The model under review builds one solid part; all positions refer to its coordinate system, in mm. A direction names the side the tool comes from. Give positions to 0.01 mm unless a question says otherwise; leave off trailing zeros. Write item = value, one per line.
```python
from build123d import *

# Parameters (mm, degrees)
F0_W      = 100
F0_H      = 100
F1_DEPTH  = 50
F2_R      = 42.5
F3_DEPTH  = 15
F4_R      = 42.5
F5_DEPTH  = 15
F6_R      = 42.5
F7_DEPTH  = 15
F8_R      = 42.5
F9_DEPTH  = 15
F10_R     = 30
F11_DEPTH = 10
F12_R     = 30
F13_DEPTH = 10
F14_R     = 30
F15_DEPTH = 10
F16_R     = 30
F17_DEPTH = 10
F18_R     = 20
F19_DEPTH = 10
F20_R     = 20
F21_DEPTH = 10
F22_R     = 20
F23_DEPTH = 10
F24_R     = 20
F25_DEPTH = 10
F26_R     = 12.5
F27_DEPTH = 10
F28_R     = 12.5
F29_DEPTH = 10
F30_R     = 12.5
F31_DEPTH = 65.001
F32_R     = 12.5
F33_DEPTH = 65.001
F34_R     = 42.5
F35_DEPTH = 15
F36_R     = 30
F37_DEPTH = 10
F38_R     = 20
F39_DEPTH = 10
F40_R     = 12.5
F41_DEPTH = 10
F42_R     = 42.5
F43_DEPTH = 15
F44_R     = 30
F45_DEPTH = 10
F46_R     = 20
F47_DEPTH = 10
F48_R     = 12.5
F49_DEPTH = 65.001


with BuildPart() as f1:
    # F0 (on Front) → F1 (new body, symmetric)
    with BuildSketch(Plane.XZ):
        Rectangle(F0_W, F0_H)
    extrude(amount=F1_DEPTH, both=True)

    # F2 (on face) → F3 (cut)
    with BuildSketch(Plane.YZ.offset(50)):
        Circle(F2_R)
    extrude(amount=-F3_DEPTH, mode=Mode.SUBTRACT)

    # F4 (on face) → F5 (cut)
    with BuildSketch(Plane.XZ.offset(50)):
        Circle(F4_R)
    extrude(amount=-F5_DEPTH, mode=Mode.SUBTRACT)

    # F6 (on face) → F7 (cut)
    with BuildSketch(Plane(origin=(-50, 0, 0), x_dir=(0, -1, 0), z_dir=(-1, 0, 0))):
        Circle(F6_R)
    extrude(amount=-F7_DEPTH, mode=Mode.SUBTRACT)

    # F8 (on face) → F9 (cut)
    with BuildSketch(Plane(origin=(0, 50, 0), x_dir=(-1, 0, 0), z_dir=(0, 1, 0))):
        Circle(F8_R)
    extrude(amount=-F9_DEPTH, mode=Mode.SUBTRACT)

    # F10 (on face) → F11 (cut)
    with BuildSketch(Plane.XZ.offset(35)):
        Circle(F10_R)
    extrude(amount=-F11_DEPTH, mode=Mode.SUBTRACT)

    # F12 (on face) → F13 (cut)
    with BuildSketch(Plane(origin=(-35, 0, 0), x_dir=(0, -1, 0), z_dir=(-1, 0, 0))):
        Circle(F12_R)
    extrude(amount=-F13_DEPTH, mode=Mode.SUBTRACT)

    # F14 (on face) → F15 (cut)
    with BuildSketch(Plane(origin=(0, 35, 0), x_dir=(-1, 0, 0), z_dir=(0, 1, 0))):
        Circle(F14_R)
    extrude(amount=-F15_DEPTH, mode=Mode.SUBTRACT)

    # F16 (on face) → F17 (cut)
    with BuildSketch(Plane.YZ.offset(35)):
        Circle(F16_R)
    extrude(amount=-F17_DEPTH, mode=Mode.SUBTRACT)

    # F18 (on face) → F19 (cut)
    with BuildSketch(Plane.YZ.offset(25)):
        Circle(F18_R)
    extrude(amount=-F19_DEPTH, mode=Mode.SUBTRACT)

    # F20 (on face) → F21 (cut)
    with BuildSketch(Plane.XZ.offset(25)):
        Circle(F20_R)
    extrude(amount=-F21_DEPTH, mode=Mode.SUBTRACT)

    # F22 (on face) → F23 (cut)
    with BuildSketch(Plane(origin=(-25, 0, 0), x_dir=(0, -1, 0), z_dir=(-1, 0, 0))):
        Circle(F22_R)
    extrude(amount=-F23_DEPTH, mode=Mode.SUBTRACT)

    # F24 (on face) → F25 (cut)
    with BuildSketch(Plane(origin=(0, 25, 0), x_dir=(-1, 0, 0), z_dir=(0, 1, 0))):
        Circle(F24_R)
    extrude(amount=-F25_DEPTH, mode=Mode.SUBTRACT)

    # F26 (on face) → F27 (cut)
    with BuildSketch(Plane(origin=(0, 15, 0), x_dir=(-1, 0, 0), z_dir=(0, 1, 0))):
        Circle(F26_R)
    extrude(amount=-F27_DEPTH, mode=Mode.SUBTRACT)

    # F28 (on face) → F29 (cut)
    with BuildSketch(Plane.YZ.offset(15)):
        Circle(F28_R)
    extrude(amount=-F29_DEPTH, mode=Mode.SUBTRACT)

    # F30 (on face) → F31 (cut, through all)
    with BuildSketch(Plane.XZ.offset(15)):
        Circle(F30_R)
    extrude(amount=-F31_DEPTH, mode=Mode.SUBTRACT)

    # F32 (on face) → F33 (cut, through all)
    with BuildSketch(Plane(origin=(-15, 0, 0), x_dir=(0, -1, 0), z_dir=(-1, 0, 0))):
        Circle(F32_R)
    extrude(amount=-F33_DEPTH, mode=Mode.SUBTRACT)

    # F34 (on face) → F35 (cut)
    with BuildSketch(Plane.XY.offset(50)):
        Circle(F34_R)
    extrude(amount=-F35_DEPTH, mode=Mode.SUBTRACT)

    # F36 (on face) → F37 (cut)
    with BuildSketch(Plane.XY.offset(35)):
        Circle(F36_R)
    extrude(amount=-F37_DEPTH, mode=Mode.SUBTRACT)

    # F38 (on face) → F39 (cut)
    with BuildSketch(Plane.XY.offset(25)):
        Circle(F38_R)
    extrude(amount=-F39_DEPTH, mode=Mode.SUBTRACT)

    # F40 (on face) → F41 (cut)
    with BuildSketch(Plane.XY.offset(15)):
        Circle(F40_R)
    extrude(amount=-F41_DEPTH, mode=Mode.SUBTRACT)

    # F42 (on face) → F43 (cut)
    with BuildSketch(Plane(origin=(0, 0, -50), x_dir=(1, 0, 0), z_dir=(0, 0, -1))):
        Circle(F42_R)
    extrude(amount=-F43_DEPTH, mode=Mode.SUBTRACT)

    # F44 (on face) → F45 (cut)
    with BuildSketch(Plane(origin=(0, 0, -35), x_dir=(1, 0, 0), z_dir=(0, 0, -1))):
        Circle(F44_R)
    extrude(amount=-F45_DEPTH, mode=Mode.SUBTRACT)

    # F46 (on face) → F47 (cut)
    with BuildSketch(Plane(origin=(0, 0, -25), x_dir=(1, 0, 0), z_dir=(0, 0, -1))):
        Circle(F46_R)
    extrude(amount=-F47_DEPTH, mode=Mode.SUBTRACT)

    # F48 (on face) → F49 (cut, through all)
    with BuildSketch(Plane(origin=(0, 0, -15), x_dir=(1, 0, 0), z_dir=(0, 0, -1))):
        Circle(F48_R)
    extrude(amount=-F49_DEPTH, mode=Mode.SUBTRACT)


solid = f1.part
```
1. Take a section at A-A on z = 0. Count the separate pieces of the cut face and the enclosed holes in it, and give its area (3 significant figures).
Findings below:
separate_pieces = 16
enclosed_holes = 0
area = 450 mm²
2. Insertion check: P1, Ø15, axis at y = 5, z = 6.5, coming from the -X side; P2, Ø5, axis at x = -5, y = 39, coming from the -Z side; P3, Ø10, axis at y = 21, z = 2.5, coming from the +X side; P4, Ø10, axis at y = 26, z = 22, coming from the +X side. Each pin has a flat end and moves straight along its axis. Give the tip position at first contact, or say it passes through.
Findings below:
P1 = -15
P2 = through
P3 = 25
P4 = 35
3. Machinability: for faces 4 (the cylindrical face through (-31.181, -16.128, 25.296)), 5 (the cylindrical face through (-5.53, 42.14, 44.27)), 6 (the flat face through (-13, 15, 0)), 7 (the cylindrical face through (-19.98, -0.88, -21.18)), which of the approach directions +Z, -Z, +X, -X, +Y, -Y give a long, thin tool a straight path to every point of the face, cutting with its end or side? Answer none if there is none.
Findings below:
face_4 = -X
face_5 = +Z
face_6 = +Y
face_7 = -Z
4. For line 1 (X direction, y = 13.75, z = 0); line 2 (Z direction, x = 1, y = -24.5), list the stretches that pass through material, from the lowest coordinate up. Write a range as from..to.
Findings below:
line_1 = -15..-12.5, 12.5..15
line_2 = -25..-19.97, 19.97..25
5. Draft analysis for pull direction Z (two halves, no side actions). For faces 1 (the cylindrical face through (-44.27, 5.53, 42.14)), 2 (the flat face through (-45, -1, 50)), 3 (the flat face through (31, 0, -35)), state which applies: +Z half, -Z half, draft (parallel to the pull), parting line (faces both ways), or undercut.
Findings below:
face_1 = undercut
face_2 = +Z half
face_3 = -Z half
